```python
from build123d import *

# Parameters (mm, degrees)
F0_W     = 838.2
F0_H     = 55.5625
F1_DEPTH = 19.05
F2_R     = 55.56249
F4_DEPTH = 55.5635
F5_R     = 9.525
F6_DEPTH = 25.4


# Not quite as in the source:
# - a fillet or chamfer is up to 0.001 mm smaller than in the source, because OpenCascade refuses the exact size


with BuildPart() as f1:
    # F0 (on Right) → F1 (new body)
    with BuildSketch(Plane.YZ):
        Rectangle(F0_W, F0_H)
    extrude(amount=F1_DEPTH)

    # F2 (radius 55.5625 in the source; OpenCascade refuses exactly that, so slightly less here)
    f2_edges = [f1.edges().sort_by_distance(p)[0] for p in [
        (9.525, 419.1, -27.78125),
    ]]
    fillet(f2_edges, radius=F2_R)

    # F3 (on face) → F4 (cut, through all)
    with BuildSketch(Plane.XY.offset(27.78125)):
        Polygon((0, -419.1), (19.05, -419.1), (0, -400.05), align=None)
    extrude(amount=-F4_DEPTH, mode=Mode.SUBTRACT)

    # F5 (on face) → F6 (cut)
    with BuildSketch(Plane.YZ.offset(19.05)):
        with Locations((391.31875, 0)):
            Circle(F5_R)
    extrude(amount=-F6_DEPTH, mode=Mode.SUBTRACT)


solid = f1.part
```
Input: part model. Units: mm. Frame: model coordinates. Coordinates: 2 decimals unless noted, no trailing zeros. Loops run counter-clockwise (first coordinate to the right, second up) from the corner with the lowest first, then second, coordinate; pieces in that order, holes last. Notation, with made-up numbers: M 7,-9.75 L 55,-9.75 A23 cw 55,13.25 Z; hole C 39,41 d11. An arc over 180 degrees is marked long. One line per item, written item: value.
(1) Line query: line 1 along Y through (x, z) = (11, -1); line 2 along Y through (x, z) = (3.25, 8.5); line 3 along Y through (x, z) = (10.25, 23.5). Output: solid intervals per line, ascending. Write a range as from..to.
Filled in:
line 1: -411.05..381.85, 400.79..411.06
line 2: -403.3..387.02, 395.62..415.65
line 3: -410.3..418.93
(2) Section B-B (z = 0). Output: boundary loops of the cut face in (x, y).
Filled in:
outline: M 0,-400.05 L 19.05,-419.1 L 19.05,381.79 L 0,381.79 Z; M 0,400.84 L 19.05,400.84 L 19.05,411.66 L 0,411.66 Z
(3) Pull-direction query (Z, two-part tool) for faces 1 (the cylindrical face through (9.66, 402.39, -11.94)), 2 (the cylindrical face through (9.658, 400.404, 2.861)), 3 (the flat face through (9, -6, 27.781)); classes: +Z half, -Z half, draft (parallel to the pull), parting line (faces both ways), or undercut.
Filled in:
face 1: -Z half
face 2: undercut
face 3: +Z half
(4) Pin query (flat end, axial travel): pin 1 (1.5 mm diameter, centred on x = 10, z = 22, fed in from -Y); pin 2 (2 mm diameter, centred on x = 16, z = 12, fed in from +Y); pin 3 (2 mm diameter, centred on x = 5, z = -10, fed in from -Y). Return the tip coordinate at first contact, or that it passes through.
Filled in:
pin 1: y = -410.8
pin 2: y = 417.1
pin 3: y = -406.05
